Source: three-view drawing plus pictorial views. Frame: mm from the lowest corner of the part. A direction names the side the tool comes from. Coordinates: 2 decimals unless noted, no trailing zeros. Loops run counter-clockwise (first coordinate to the right, second up) from the corner with the lowest first, then second, coordinate; pieces in that order, holes last.
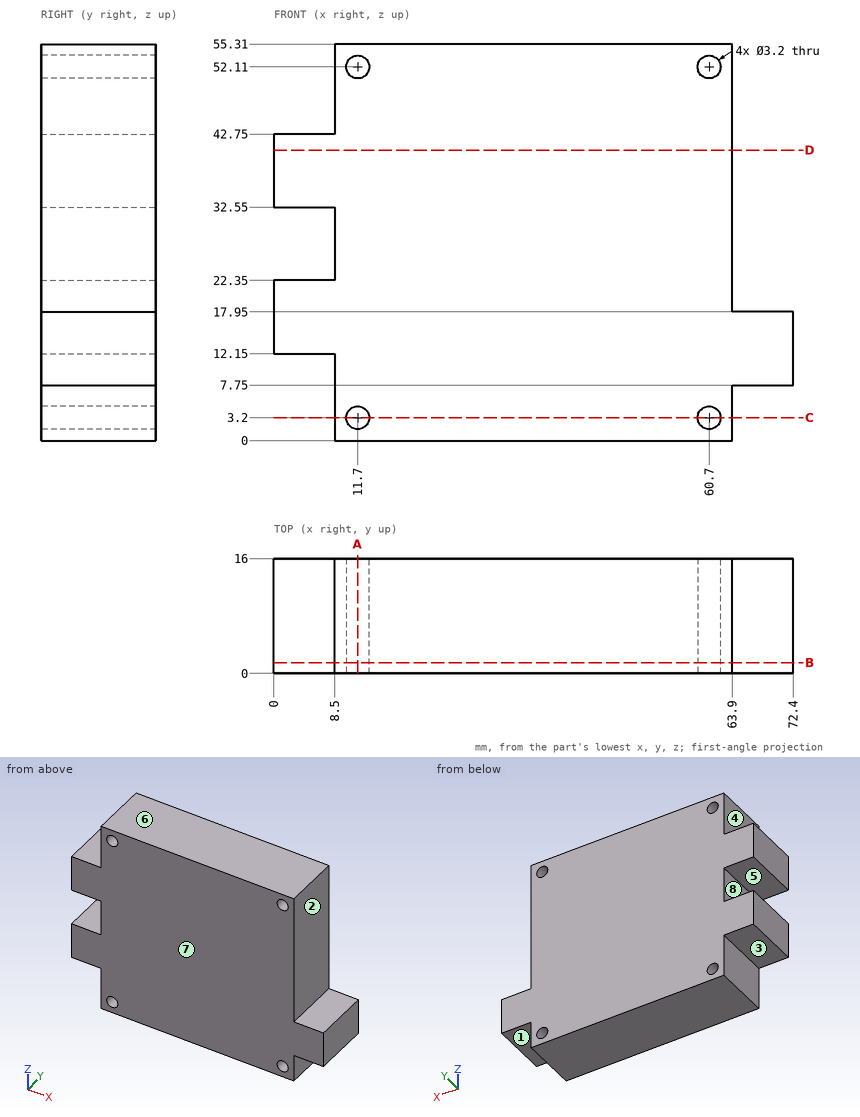
Q1. Section query C-C on z = 3.2. Return the cut outline in (x, y), then the cut area to 3 significant figures.
Q2. Material intervals for line 1 along Z through (x, y) = (11.7, 5); line 2 along X through (y, z) = (5, 52.11); line 3 along X through (y, z) = (12.75, 34), sorted ascending.
Q3. Section query A-A on x = 11.7. Return the cut outline in (y, z).
Q4. First-contact query: pin 1 Ø8 at (y, z) = (5.5, 36) entering from +X; pin 2 Ø3 at (x, z) = (11.7, 52.11) entering from +Y; pin 3 Ø7 at (x, y) = (4, 5.5) entering from -Z; pin 4 Ø9.5 at (y, z) = (11, 5.5) entering from -X. Flat tips, straight axial feed; report the tip coordinate or a pass-through.
Q5. Section query D-D on z = 40.5. Return the cut outline in (x, y), then the cut area to 3 significant figures.
Q6. Section query B-B on y = 1.5. Return the cut outline in (x, z).
Q7. Reachability of the marked faces 1, 2, 3, 4 and 5 from +Z, -Z, +X, -X, +Y, -Y: full face, straight path, thin tool, end or side. Return the list, or none.
Q8. Draft query along Z for the marked faces 6, 7 and 8. Return one class per face: released by +Z, released by -Z, zero draft, split by the parting line, or undercut.
Resolved:
1. outline: (8.5, 0) - (10.1, 0) - (10.1, 16) - (8.5, 16) - close; (13.3, 0) - (59.1, 0) - (59.1, 16) - (13.3, 16) - close; (62.3, 0) - (63.9, 0) - (63.9, 16) - (62.3, 16) - close
1. area: 784 mm2
2. line 1: z = 0 to 1.6, 4.8 to 50.51, 53.71 to 55.31
2. line 2: x = 8.5 to 10.1, 13.3 to 59.1, 62.3 to 63.9
2. line 3: x = 0 to 63.9
3. outline: (0, 0) - (16, 0) - (16, 1.6) - (0, 1.6) - close; (0, 4.8) - (16, 4.8) - (16, 50.51) - (0, 50.51) - close; (0, 53.71) - (16, 53.71) - (16, 55.31) - (0, 55.31) - close
4. pin 1: stops at x = 63.9
4. pin 2: passes through
4. pin 3: stops at z = 12.15
4. pin 4: stops at x = 8.5
5. outline: (0, 0) - (63.9, 0) - (63.9, 16) - (0, 16) - close
5. area: 1,020 mm2
6. outline: (0, 12.15) - (8.5, 12.15) - (8.5, 0) - (63.9, 0) - (63.9, 7.75) - (72.4, 7.75) - (72.4, 17.95) - (63.9, 17.95) - (63.9, 55.31) - (8.5, 55.31) - (8.5, 42.75) - (0, 42.75) - (0, 32.55) - (8.5, 32.55) - (8.5, 22.35) - (0, 22.35) - close; hole circle Ø3.2 at (11.7, 3.2); hole circle Ø3.2 at (11.7, 52.11); hole circle Ø3.2 at (60.7, 3.2); hole circle Ø3.2 at (60.7, 52.11)
7. face 1: -Z, +X, +Y, -Y
7. face 2: +Z, +X, +Y, -Y
7. face 3: -Z, -X, +Y, -Y
7. face 4: +Z, -X, +Y, -Y
7. face 5: -X, +Y, -Y
8. face 6: released by +Z
8. face 7: zero draft
8. face 8: undercut
